```python
from build123d import *

# Parameters (mm, degrees)
SKETCH1_R                           = 36.195
BOSS_EXTRUDE1_DEPTH                 = 7
CUT_EXTRUDE1_REACH                  = 53.664
SKETCH2_R                           = 6.35
BOSS_EXTRUDE2_DEPTH                 = 68.58
FILLET1_R                           = 2.54
F_9_64_0_14063_DIAMETER_HOLE1_D     = 3.572002
F_9_64_0_14063_DIAMETER_HOLE1_DEPTH = 5.5999888
F_9_64_0_14063_DIAMETER_HOLE1_TIP   = 1.073137666
F_9_64_0_14063_DIAMETER_HOLE2_D     = 3.572002
F_9_64_0_14063_DIAMETER_HOLE2_DEPTH = 5.588
F_9_64_0_14063_DIAMETER_HOLE2_TIP   = 1.073137666


with BuildPart() as part:
    # Sketch1 → Boss-Extrude1 (new body)
    with BuildSketch(Plane(origin=(0, 0, 0), x_dir=(1, 0, 0), z_dir=(0, 1, 0))):
        with Locations(Location((0, 0, 0), (0, 0, 270))):
            Circle(SKETCH1_R)
    extrude(amount=-BOSS_EXTRUDE1_DEPTH)

    # Sketch2 → Cut-Extrude1 (cut, up to next)
    with BuildSketch(Plane.XZ.offset(7), mode=Mode.PRIVATE) as cut_extrude1_sk1:
        with Locations(Location((0, 0, 0), (0, 0, 270))):
            Circle(SKETCH2_R)
    cut_extrude1_tool1 = extrude(cut_extrude1_sk1.sketch, amount=-CUT_EXTRUDE1_REACH, mode=Mode.PRIVATE) & part.part
    add(cut_extrude1_tool1.solids().sort_by_distance((0, -7, 0))[0], mode=Mode.SUBTRACT)

    # Sketch3 → Boss-Extrude2 (add)
    with BuildSketch(Plane(origin=(0, 0, 0), x_dir=(1, 0, 0), z_dir=(0, 1, 0))):
        Polygon((0, 24.929984624), (-21.59, -12.464992312), (21.59, -12.464992312), align=None)
        Polygon((12.791181898, -7.384992312), (0, 14.769984624), (-12.791181898, -7.384992312), align=None, mode=Mode.SUBTRACT)
    extrude(amount=BOSS_EXTRUDE2_DEPTH)

    # Fillet1
    fillet1_edges = [part.edges().sort_by_distance(p)[0] for p in [
        (21.59, 34.29, 12.464992312),
        (0, 34.29, -24.929984624),
        (-21.59, 34.29, 12.464992312),
        (12.791181898, 34.29, 7.384992312),
        (0, 34.29, -14.769984624),
        (-12.791181898, 34.29, 7.384992312),
    ]]
    fillet(fillet1_edges, radius=FILLET1_R)

    # 9_64 _0.14063_ Diameter Hole1
    with Locations(Plane.XY.offset(12.464992312)):
        with Locations((-11.5, 61.5), (11.5, 61.5), (-11.5, 3.5), (11.5, 3.5)):
            Hole(F_9_64_0_14063_DIAMETER_HOLE1_D / 2, depth=F_9_64_0_14063_DIAMETER_HOLE1_DEPTH)
            with Locations((0, 0, -(F_9_64_0_14063_DIAMETER_HOLE1_DEPTH + F_9_64_0_14063_DIAMETER_HOLE1_TIP / 2))):  # 118° drill point
                Cone(0, F_9_64_0_14063_DIAMETER_HOLE1_D / 2, F_9_64_0_14063_DIAMETER_HOLE1_TIP, mode=Mode.SUBTRACT)

    # 9_64 _0.14063_ Diameter Hole2
    with Locations(Plane(origin=(0, -7, 0), x_dir=(-1, 0, 0), z_dir=(0, -1, 0))):
        with Locations((-19.05, 0), (19.05, 0)):
            Hole(F_9_64_0_14063_DIAMETER_HOLE2_D / 2, depth=F_9_64_0_14063_DIAMETER_HOLE2_DEPTH)
            with Locations((0, 0, -(F_9_64_0_14063_DIAMETER_HOLE2_DEPTH + F_9_64_0_14063_DIAMETER_HOLE2_TIP / 2))):  # 118° drill point
                Cone(0, F_9_64_0_14063_DIAMETER_HOLE2_D / 2, F_9_64_0_14063_DIAMETER_HOLE2_TIP, mode=Mode.SUBTRACT)


solid = part.part
```
Geometry check sheet. Reference: the model listing, model coordinates, mm. A direction names the side the tool comes from. Coordinates: 2 decimals unless noted, no trailing zeros. Loops run counter-clockwise (first coordinate to the right, second up) from the corner with the lowest first, then second, coordinate; pieces in that order, holes last. Notation, with made-up numbers: (-10, -4) - (48, -4) arc R17 ccw to (48, 8) - close; hole circle Ø3 at (73, 19.5). An arc over 180 degrees is marked (long way). One line per item, written item: value. Start each with the question number.
(1) Cross-section at D-D on z = -7.5. Enter the section's corners in (x, y).
(2) Depth check by flat-ended pin: P1, Ø5, axis at y = 29, z = -17.5, coming from the +X side; P2, Ø3, axis at x = 11.5, y = 3.5, coming from the +Z side; P3, Ø4, axis at y = 10, z = 10, coming from the -X side. Enter the tip coordinate at first touch or a pass-through.
(3) Tool access check on faces 5 (the cylindrical face through (19.37, 34.77, 11.23)), 6 (the flat face through (0, 34, 7.385)), 7 (the cylindrical face through (-0.04, 34.77, -22.39)), 8 (the cylindrical face through (12.917, 2.413, 9.626)), 9 (the cylindrical face through (-20.834, -4.167, -0.079)). Record the directions out of +Z, -Z, +X, -X, +Y, -Y that give a thin tool (end or side, any length) a straight path to the whole face; none if there is none.
(4) Cross-section at A-A on y = 12.5. Enter the section's corners in (x, z) (3 decimals).
(5) Cross-section at B-B on x = 0. Enter the section's corners in (y, z) (3 decimals).
(6) Cross-section at C-C on x = 16. Enter the section's corners in (y, z) (3 decimals).
(7) Mould release check, pull along X, two halves, no side actions. Record for faces 1 (the cylindrical face through (17.266, -4.167, -0.079)), 2 (the conical face through (11.8, 3.59, 5.98)), 3 (the cylindrical face through (-19.41, 34.77, 11.16)), 4 (the flat face through (8.5, 68.58, -1.3)): released by +X, released by -X, zero draft, split by the parting line, or undercut.
(8) Material ranges on line 1 (X direction, y = 61.5, z = 9.5); line 2 (X direction, y = 61.5, z = 9.1); line 3 (Y direction, x = -11, z = 11), recorded low to high. Write a range as [from, to].
Results below:
1. outline: (-35.41, -7) - (35.41, -7) - (35.41, 0) - (10.06, 0) - (10.06, 68.58) - (4.2, 68.58) - (4.2, 0) - (-4.2, 0) - (-4.2, 68.58) - (-10.06, 68.58) - (-10.06, 0) - (-35.41, 0) - close
2. P1: stops at x = 5.73
2. P2: stops at z = 6.69
2. P3: stops at x = -19.73
3. face 5: +X, +Y
3. face 6: +Y
3. face 7: -Z, +Y
3. face 8: +Z
3. face 9: -Y
4. outline: (-19.39, 8.655) - (-2.2, -21.12) arc R2.54 ccw to (2.2, -21.12) - (19.39, 8.655) arc R2.54 ccw to (17.191, 12.465) - (-17.191, 12.465) arc R2.54 ccw to start; hole (-10.591, 3.575) - (-2.2, -10.96) arc R2.54 ccw to (2.2, -10.96) - (10.591, 3.575) arc R2.54 ccw to (8.392, 7.385) - (-8.392, 7.385) arc R2.54 ccw to start
5. outline: (-7, -36.195) - (0, -36.195) - (0, -22.39) - (68.58, -22.39) - (68.58, -12.23) - (0, -12.23) - (0, -6.35) - (-7, -6.35) - close; (-7, 6.35) - (0, 6.35) - (0, 7.385) - (68.58, 7.385) - (68.58, 12.465) - (0, 12.465) - (0, 36.195) - (-7, 36.195) - close
6. outline: (-7, -32.467) - (0, -32.467) - (0, 2.783) - (68.58, 2.783) - (68.58, 12.465) - (0, 12.465) - (0, 32.467) - (-7, 32.467) - close
7. face 1: undercut
7. face 2: undercut
7. face 3: released by -X
7. face 4: zero draft
8. line 1: x = [-19.69, -13.29], [-9.71, 9.71], [13.29, 19.69]
8. line 2: x = [-19.59, -13.29], [-9.71, 9.71], [13.29, 19.59]
8. line 3: y = [-7, 1.79], [5.21, 59.79], [63.21, 68.58]
